Geometry check sheet. Reference: the model listing, model coordinates, mm. Give positions to 0.01 mm unless a question says otherwise; leave off trailing zeros. Order: outer loops, then holes, each group sorted by start corner. A loop starts at its lowest first (then second) coordinate and runs counter-clockwise, first axis right, second up. Notation, with made-up numbers: (-34.5, -33) - (15.5, -33) arc R20 cw to (15.5, -15) - close; hole circle Ø4 at (-36, 58). An arc over 180 degrees is marked (long way). Put each result on its own line as item: value. Start each with the question number.
```python
from build123d import *

# Parameters (mm, degrees)
F0_R     = 7.3025
F0_R_2   = 6.35
F1_DEPTH = 1.5875
F2_R     = 0.4445


with BuildPart() as f1:
    # F0 (on Front) → F1 (new body, symmetric)
    with BuildSketch(Plane.XZ):
        Circle(F0_R)
        Circle(F0_R_2, mode=Mode.SUBTRACT)
    extrude(amount=F1_DEPTH, both=True)

    # F2
    f2_edges = [f1.edges().sort_by_distance(p)[0] for p in [
        (-7.3025, -1.5875, 0),
        (-6.35, -1.5875, 0),
        (-7.3025, 1.5875, 0),
        (-6.35, 1.5875, 0),
    ]]
    fillet(f2_edges, radius=F2_R)

    # F3 (on Front) → F4 (revolve)
    with BuildSketch(Plane.XZ):
        Polygon((0, 9.3345), (0, 6.7945), (1.670926, 9.3345), align=None)
    revolve(axis=Axis((0, 0, 8.0645), (0, 0, 1)))

    # F5 (on Front) → F6 (revolve, cut)
    with BuildSketch(Plane.XZ):
        Polygon((1.410544, 9.829888), (0, 9.829888), (0, 7.456552), align=None)
    revolve(axis=Axis((0, 0, 8.64322), (0, 0, 1)), mode=Mode.SUBTRACT)


solid = f1.part
```
Item 1: Cross-section at B-B (y = 0.6). Count the separate pieces of the cut face and the enclosed holes in it, and give its area (3 significant figures).
Item 2: Thickness scan on line 1 along Z through (x, y) = (0, 0.5); line 2 along Z through (x, y) = (0, 0.1); line 3 along Z through (x, y) = (0, 0.3). Record the ranges inside material, lowest first.
Item 3: Release check for a two-part mould opening along Y. For faces 1 (the face through (-1.38, 0.02, -6.2)), 2 (the face through (-0.1, -0.43, 8.2)) record: +Y half, -Y half, draft (parallel to the pull), parting line (faces both ways), or undercut.
Item 4: Gauge pin test, flat ends, axial feed: pin 1 Ø1 at (x, y) = (-3.5, 0) entering from +Z; pin 2 Ø1.5 at (y, z) = (0, 5) entering from -X; pin 3 Ø1 at (x, y) = (-2, -1) entering from +Z. Record the tip position at first contact, or that the pin passes through.
Item 5: Cross-section at A-A (z = 0). Enter the section's corners in (x, y).
Recorded:
1. separate pieces: 2
1. enclosed holes: 1
1. area: 42.9 mm^2
2. line 1: z = -7.3 to -6.35, 6.35 to 7.3, 7.55 to 8.3
2. line 2: z = -7.3 to -6.35, 6.35 to 7.62
2. line 3: z = -7.3 to -6.35, 6.35 to 7.96
3. face 1: draft
3. face 2: undercut
4. pin 1: stops at z = 6.66
4. pin 2: stops at x = -5.94
4. pin 3: stops at z = 7.15
5. outline: (-7.3, -1.14) arc R0.44 ccw to (-6.86, -1.59) - (-6.79, -1.59) arc R0.44 ccw to (-6.35, -1.14) - (-6.35, 1.14) arc R0.44 ccw to (-6.79, 1.59) - (-6.86, 1.59) arc R0.44 ccw to (-7.3, 1.14) - close; (6.35, -1.14) arc R0.44 ccw to (6.79, -1.59) - (6.86, -1.59) arc R0.44 ccw to (7.3, -1.14) - (7.3, 1.14) arc R0.44 ccw to (6.86, 1.59) - (6.79, 1.59) arc R0.44 ccw to (6.35, 1.14) - close
